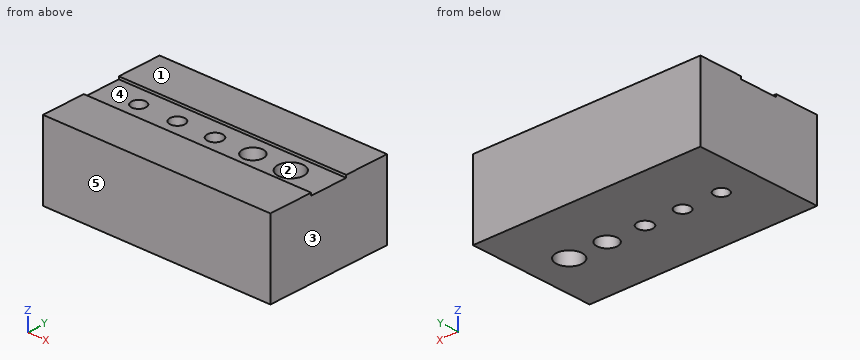
```python
from build123d import *

# Parameters (mm, degrees)
F0_W     = 57.15
F0_H     = 11.1125
F0_H_2   = 9.525
F0_R     = 1.778
F0_R_2   = 1.8415
F0_R_3   = 1.905
F0_R_4   = 2.54
F0_R_5   = 3.175
F1_DEPTH = 19.05
F2_DEPTH = 0.635


with BuildPart() as f1:
    # F0 (on Top) → F1 (new body)
    with BuildSketch(Plane.XY):
        with Locations((0, 10.31875)):
            Rectangle(F0_W, F0_H)
        Rectangle(F0_W, F0_H_2)
        with Locations((-19.177, 0)):
            Circle(F0_R, mode=Mode.SUBTRACT)
        with Locations((-9.4615, 0)):
            Circle(F0_R_2, mode=Mode.SUBTRACT)
        Circle(F0_R_3, mode=Mode.SUBTRACT)
        with Locations((9.525, 0)):
            Circle(F0_R_4, mode=Mode.SUBTRACT)
        with Locations((19.05, 0)):
            Circle(F0_R_5, mode=Mode.SUBTRACT)
        with Locations((0, -10.31875)):
            Rectangle(F0_W, F0_H)
    extrude(amount=-F1_DEPTH)

    # F0 (on Top) → F2 (cut)
    with BuildSketch(Plane.XY):
        Rectangle(F0_W, F0_H_2)
        with Locations((-19.177, 0)):
            Circle(F0_R, mode=Mode.SUBTRACT)
        with Locations((-9.4615, 0)):
            Circle(F0_R_2, mode=Mode.SUBTRACT)
        Circle(F0_R_3, mode=Mode.SUBTRACT)
        with Locations((9.525, 0)):
            Circle(F0_R_4, mode=Mode.SUBTRACT)
        with Locations((19.05, 0)):
            Circle(F0_R_5, mode=Mode.SUBTRACT)
    extrude(amount=-F2_DEPTH, mode=Mode.SUBTRACT)


solid = f1.part
```
Check sheet for the modelled part. Datum: model origin and axes. Units: mm. Face numbers are marked on the shaded views. A direction names the side the tool comes from. Give positions to 0.01 mm unless a question says otherwise; leave off trailing zeros. Write each loop counter-clockwise with the first axis right and the second up, starting at its lowest first coordinate (ties: lowest second). Pieces come first, ordered by that corner, then holes.
Item 1: Draft check along X on the marked faces 1, 2 and 3. Enter one of: released by +X, released by -X, zero draft, split by the parting line, or undercut.
Item 2: Cross-section at C-C (z = -9.75). Count the separate pieces of the cut face and the enclosed holes in it, and give its area (3 significant figures).
Item 3: Scan lines: L1, parallel to X at y = -2, z = -16 (3 decimals); L2, parallel to Y at x = 16.5, z = -17.25 (3 decimals); L3, parallel to Z at x = 3, y = -2.5 (3 decimals). Record each from-to range of solid material in increasing order.
Item 4: Cross-section at B-B (y = 0). Enter the section's corners in (x, z) (3 decimals).
Item 5: Access from +Z, -Z, +X, -X, +Y, -Y to the whole of each face (thin tool, end or side, straight path). Record for the marked faces 4 and 5.
Item 6: Gauge pin test, flat ends, axial feed: pin 1 (4 mm diameter, centred on x = 19.05, y = 0, fed in from -Z); pin 2 (10 mm diameter, centred on x = 8.5, y = 7, fed in from +Z); pin 3 (5 mm diameter, centred on x = 0, y = 0, fed in from +Z) (3 decimals). Record the tip position at first contact, or that the pin passes through.
Report:
1. face 1: zero draft
1. face 2: undercut
1. face 3: released by +X
2. separate pieces: 1
2. enclosed holes: 5
2. area: 1,730 mm2
3. L1: x = -28.575 to 7.959, 11.091 to 16.584, 21.516 to 28.575
3. L2: y = -15.875 to -1.892, 1.892 to 15.875
3. L3: z = -19.05 to -0.635
4. outline: (-28.575, -19.05) - (-20.955, -19.05) - (-20.955, -0.635) - (-28.575, -0.635) - close; (-17.399, -19.05) - (-11.303, -19.05) - (-11.303, -0.635) - (-17.399, -0.635) - close; (-7.62, -19.05) - (-1.905, -19.05) - (-1.905, -0.635) - (-7.62, -0.635) - close; (1.905, -19.05) - (6.985, -19.05) - (6.985, -0.635) - (1.905, -0.635) - close; (12.065, -19.05) - (15.875, -19.05) - (15.875, -0.635) - (12.065, -0.635) - close; (22.225, -19.05) - (28.575, -19.05) - (28.575, -0.635) - (22.225, -0.635) - close
5. face 4: +Z, +X, -X
5. face 5: +Z, -Z, +X, -X, -Y
6. pin 1: passes through
6. pin 2: stops at z = 0
6. pin 3: stops at z = -0.635
